from build123d import *

# Parameters (mm, degrees)
F0_W     = 68.784848
F0_H     = 128.761858
F1_DEPTH = 2.54
F2_DEPTH = 17.78


with BuildPart() as f1:
    # F0 (on Front) → F1 (new body)
    with BuildSketch(Plane.XZ):
        Rectangle(F0_W, F0_H)
    extrude(amount=F1_DEPTH)

    # F0 (on Front) → F2 (join)
    with BuildSketch(Plane.XZ):
        Polygon((34.392424, -64.380929), (-34.392424, -64.380929), (-34.392424, -75.285852), (34.811836, -75.285852), (34.811836, -64.380929), align=None)
    extrude(amount=F2_DEPTH)


solid = f1.part
Work out the finished part from the listing and answer in its coordinate system (mm). A direction names the side the tool comes from. Give positions to 0.01 mm unless a question says otherwise; leave off trailing zeros. Loops run counter-clockwise (first coordinate to the right, second up) from the corner with the lowest first, then second, coordinate; pieces in that order, holes last. Notation, with made-up numbers: (-4, 31) - (15, 31) arc R20 cw to (15, 54) - close; hole circle Ø2 at (-6.5, 25.25). An arc over 180 degrees is marked (long way). Answer in a Markdown table with one row per item. Add a question column.
Q1. The part is cut by section A-A (y = -5.25). Determine the outline of the cut face in (x, z), and give its area (3 significant figures).
Q2. Consider line 1 along Z through (x, y) = (8.5, -13.25); line 2 along Y through (x, z) = (-16.5, -15.5); line 3 along X through (y, z) = (-0.75, -40). Determine where each line is inside the solid, lowest interval first.
Q3. The part is cut by section C-C (z = 34.5). Determine the outline of the cut face in (x, y), and give its area (3 significant figures).
Q4. Each of these flat-tipped pins is pushed along its axis until it touches: P1, Ø9, axis at x = 8.5, y = -12, coming from the +Z side; P2, Ø2, axis at y = -4, z = 39, coming from the -X side; P3, Ø2, axis at y = -1.5, z = -22.5, coming from the +X side. Where does it stop, or does it pass through?
Q5. The part is cut by section B-B (x = 13). Determine the outline of the cut face in (y, z), and give its area (3 significant figures).
Q6. A tool of negligible diameter and unlimited length cuts with its end or side. For faces 1 (the flat face through (-34.392, -2, -26)), 2 (the flat face through (0, -2.54, 1)), 3 (the flat face through (34.392, -1, -1)), from which of +Z, -Z, +X, -X, +Y, -Y can it reach the whole face along a straight path? Write none if from no direction.
Solution:
| question | item | result |
|---|---|---|
| 1 | outline | (-34.39, -75.29) - (34.81, -75.29) - (34.81, -64.38) - (-34.39, -64.38) - close |
| 1 | area | 755 mm² |
| 2 | line 1 | z = -75.29 to -64.38 |
| 2 | line 2 | y = -2.54 to 0 |
| 2 | line 3 | x = -34.39 to 34.39 |
| 3 | outline | (-34.39, -2.54) - (34.39, -2.54) - (34.39, 0) - (-34.39, 0) - close |
| 3 | area | 175 mm² |
| 4 | P1 | stops at z = -64.38 |
| 4 | P2 | passes through |
| 4 | P3 | stops at x = 34.39 |
| 5 | outline | (-17.78, -75.29) - (0, -75.29) - (0, 64.38) - (-2.54, 64.38) - (-2.54, -64.38) - (-17.78, -64.38) - close |
| 5 | area | 521 mm² |
| 6 | face 1 | +Z, -Z, -X, +Y, -Y |
| 6 | face 2 | +Z, +X, -X, -Y |
| 6 | face 3 | +Z, +X, +Y, -Y |
